Input: part model. Units: mm. Frame: model coordinates. Coordinates: 2 decimals unless noted, no trailing zeros. Loops run counter-clockwise (first coordinate to the right, second up) from the corner with the lowest first, then second, coordinate; pieces in that order, holes last.
(1) Line query: L1, parallel to Y at x = -113.5, z = 4.75; L2, parallel to X at y = 37, z = 4.5; L3, parallel to Y at x = -20, z = 4.5. Output: solid intervals per line, ascending.
(2) Section D-D, the plane x = -80. Return loops of the section in (y, z).
(3) Contact query for flat-ended pins moving along their axis: P1, Ø2, axis at x = -35.5, z = 4, coming from the +Y side; P2, Ø1, axis at y = 55.5, z = 6, coming from the -X side; P3, Ø1.5, axis at x = -98.5, z = 5, coming from the +Y side. Output: stop coordinate, or through.
(4) Section C-C, the plane z = 3. Give the number of separate pieces and of enclosed holes in the cut face, then the cut area to 3 significant figures.
(5) Section B-B, the plane x = -20. Return loops of the section in (y, z).
(6) Section A-A, the plane x = -149.5. Return loops of the section in (y, z).
```python
from build123d import *

# Parameters (mm, degrees)
F1_DEPTH = 6.5
F3_D     = 8.3


with BuildPart() as f1:
    # F0 (on Top) → F1 (new body)
    with BuildSketch(Plane.XY):
        Polygon((-259.8076211353, 0), (0, 0), (0, 150), align=None)
    extrude(amount=F1_DEPTH)

    # F3 (through all)
    with Locations(Plane.XY.offset(6.5)):
        with Locations((-80, 80.7179676972), (-114.6410161514, 60.7179676972), (-80, 34.5299461621), (-20, 115.3589838486), (-20, 75.3589838486), (-20, 35.3589838486), (-114.6410161514, 14.5299461621), (-149.2820323028, 40.7179676972), (-183.9230484541, 20.7179676972)):
            Hole(F3_D / 2)


solid = f1.part
```
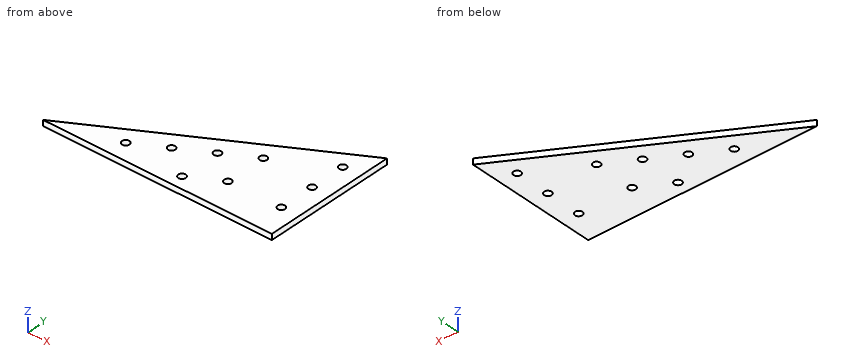
Report:
1. L1: y = 0 to 10.54, 18.52 to 56.73, 64.71 to 84.47
1. L2: x = -195.72 to -151.13, -147.44 to -83.33, -76.67 to -23.81, -16.19 to 0
1. L3: y = 0 to 31.21, 39.51 to 71.21, 79.51 to 111.21, 119.51 to 138.45
2. outline: (0, 0) - (30.38, 0) - (30.38, 6.5) - (0, 6.5) - close; (38.68, 0) - (76.57, 0) - (76.57, 6.5) - (38.68, 6.5) - close; (84.87, 0) - (103.81, 0) - (103.81, 6.5) - (84.87, 6.5) - close
3. P1: stops at y = 130.08
3. P2: stops at x = -164.54
3. P3: stops at y = 93.56
4. separate pieces: 1
4. enclosed holes: 9
4. area: 19,000 mm2
5. outline: (0, 0) - (31.21, 0) - (31.21, 6.5) - (0, 6.5) - close; (39.51, 0) - (71.21, 0) - (71.21, 6.5) - (39.51, 6.5) - close; (79.51, 0) - (111.21, 0) - (111.21, 6.5) - (79.51, 6.5) - close; (119.51, 0) - (138.45, 0) - (138.45, 6.5) - (119.51, 6.5) - close
6. outline: (0, 0) - (36.57, 0) - (36.57, 6.5) - (0, 6.5) - close; (44.86, 0) - (63.69, 0) - (63.69, 6.5) - (44.86, 6.5) - close
